Job drawing, mm, ordinate dimensions from the low corner. One solid piece. A direction names the side the tool comes from. Coordinates: 2 decimals unless noted, no trailing zeros. Order: outer loops, then holes, each group sorted by start corner. A loop starts at its lowest first (then second) coordinate and runs counter-clockwise, first axis right, second up. Notation, with made-up numbers: (-13.75, 44) - (-6.75, 44) arc R9 ccw to (-6.75, 49) - close; hole circle Ø6 at (52.5, 40.25). An arc over 180 degrees is marked (long way). Use one line per item in the form item = value.
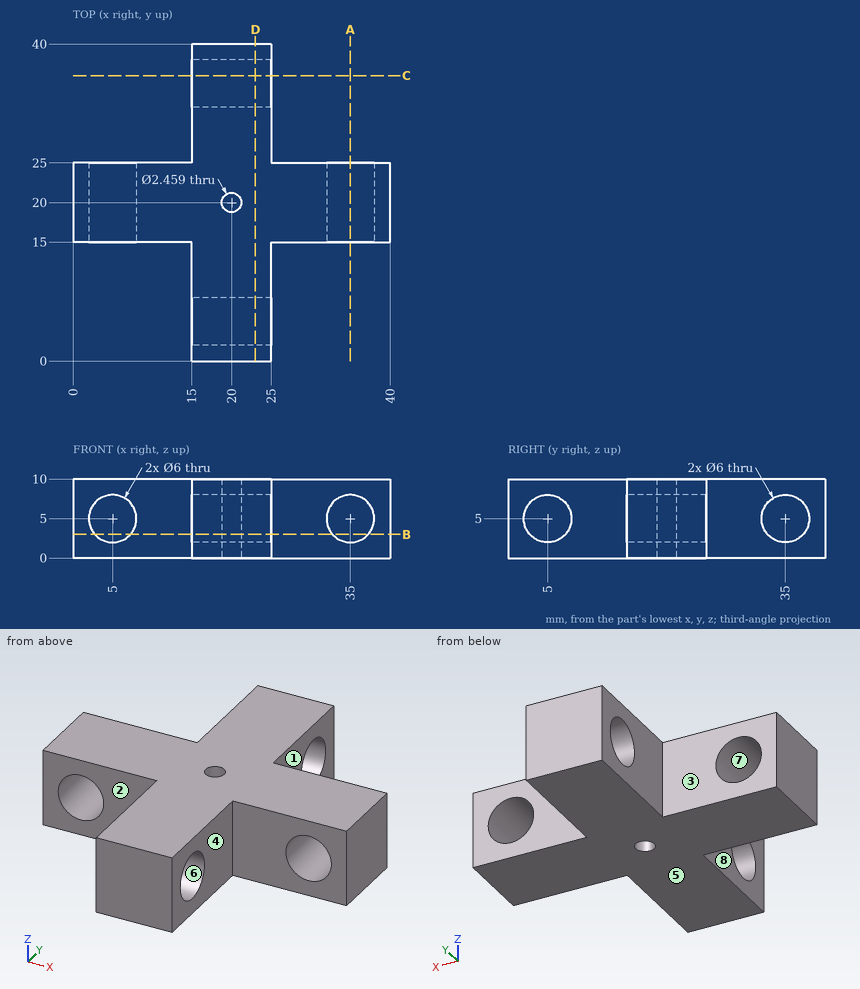
Item 1: Drill centre lines: line 1 (Y direction, x = 22.5, z = 5); line 2 (Y direction, x = 20, z = 5); line 3 (Z direction, x = 5, y = 21.25). Where is each one in solid material? Low to high. Write a range as [from, to].
Derived:
line_1 = [0, 2], [8, 32], [38, 40]
line_2 = [0, 2], [8, 18.77], [21.23, 32], [38, 40]
line_3 = [0, 2], [8, 10]
Item 2: Cut at D-D, the plane x = 23. Write the cut outline in (y, z).
Derived:
outline = (0, 0) - (40, 0) - (40, 10) - (0, 10) - close; hole circle Ø6 at (5, 5); hole circle Ø6 at (35, 5)
Item 3: Cut at A-A, the plane x = 35. Write the cut outline in (y, z), plus the area to 3 significant figures.
Derived:
outline = (15, 0) - (25, 0) - (25, 2) - (15, 2) - close; (15, 8) - (25, 8) - (25, 10) - (15, 10) - close
area = 40.0 mm²
Item 4: Cut at C-C, the plane y = 36. Write the cut outline in (x, z), plus the area to 3 significant figures.
Derived:
outline = (15, 0) - (25, 0) - (25, 2.17) - (15, 2.17) - close; (15, 7.83) - (25, 7.83) - (25, 10) - (15, 10) - close
area = 43.4 mm²
Item 5: Cut at B-B, the plane z = 3. State how many separate pieces and enclosed holes the cut face has, plus the area to 3 significant figures.
Derived:
separate_pieces = 5
enclosed_holes = 1
area = 516 mm²
Item 6: 3-axis set-ups, long thin cutter, end or side, ignore diameter. For the marked faces 1, 2, 3 and 4: which of +Z, -Z, +X, -X, +Y, -Y reach the whole face in a straight line?
Derived:
face_1 = +Z, -Z, +X, +Y
face_2 = +Z, -Z, -X, -Y
face_3 = +Z, -Z, -X, +Y
face_4 = +Z, -Z, +X, -Y
Item 7: Drop flat-ended pins along their axis: pin 1 (1.5 mm diameter, centred on x = 9, z = 6.5, fed in from +Y); pin 2 (5 mm diameter, centred on x = 10.5, z = 2.5, fed in from -Y); pin 3 (3 mm diameter, centred on y = 32, z = 3.5, fed in from +X); pin 4 (5.5 mm diameter, centred on y = 35, z = 5, fed in from -X). Give the stop position or say it passes through.
Derived:
pin_1 = 25
pin_2 = 15
pin_3 = 25
pin_4 = through
Item 8: Two-plate mould, pull along Z, no slides. Class the marked faces 5, 6, 7 and 8: +Z half, -Z half, draft (parallel to the pull), parting line (faces both ways), or undercut.
Derived:
face_5 = -Z half
face_6 = undercut
face_7 = undercut
face_8 = draft
